Read the model definition and answer for the solid it produces. Units are mm, in the model's axes. A direction names the side the tool comes from. Give positions to 0.01 mm unless a question says otherwise; leave off trailing zeros. Loops run counter-clockwise (first coordinate to the right, second up) from the corner with the lowest first, then second, coordinate; pieces in that order, holes last. Notation, with made-up numbers: (60.25, 6) -> (80.25, 6) arc R17 cw to (80.25, 13) -> close; hole circle Ø10 at (-3, 62.5). An arc over 180 degrees is marked (long way). Write each question's results on one line, items separated by ' | '. Start each with the question number.
Item 1: Section B-B on x = 14.5 is taken. Write down the section's boundary in (y, z), and give its area (3 significant figures).
Item 2: Determine the mould class of faces 1 (the cylindrical face through (-17.198, 33.596, 6.261)), 2 (the conical face through (15.932, -27.797, 5.239)), 3 (the flat face through (0, 0, 0)) for opening direction Z: +Z half, -Z half, draft (parallel to the pull), parting line (faces both ways), or undercut.
Item 3: Which of the six approach directions +Z, -Z, +X, -X, +Y, -Y give full straight-line access (tool end or side, diameter ignored) to faces 4 (the flat face through (-26, -35, 6)), 5 (the cylindrical face through (-17, -33.5, 6.3)), 6 (the cylindrical face through (22.22, -15.463, 5.425)), 7 (the cylindrical face through (-22.22, 25.787, 5.425))?
Item 4: Section A-A on x = 21 is taken. Write down the section's boundary in (y, z).
Item 5: Each of these flat-tipped pins is pushed along its axis until it touches: P1, Ø3, axis at y = -27.5, z = 5.2, coming from the +X side; P2, Ø1.5, axis at x = -0.5, y = -13.5, coming from the -Z side; P3, Ø1.9, axis at y = -20.625, z = 5.2, coming from the -X side; P4, Ø3, axis at y = 20.625, z = 5.2, coming from the -X side. Where does it stop, or does it pass through?
Item 6: Find the intervals of material crossed by line 1 (Z direction, x = 23, y = 0); line 2 (X direction, y = 29.5, z = 6.5); line 3 (Y direction, x = -23, z = 9), in increasing order.
```python
from build123d import *

# Parameters (mm, degrees)
SKETCH1_W                           = 55
SKETCH1_H                           = 70
BOSS_EXTRUDE1_DEPTH                 = 12.7
SKETCH21_RX                         = 14
SKETCH21_RY                         = 10.5
CUT_EXTRUDE1_DEPTH                  = 47.287579328
FILLET2_START                       = -1
FILLET2_DEPTH                       = 15
F_8_32_TAPPED_HOLE1_AT_2_COUNT      = 2
F_8_32_TAPPED_HOLE1_AT_2_PITCH      = 13.75
F_8_32_TAPPED_HOLE1_AT_3_COUNT      = 2
F_8_32_TAPPED_HOLE1_AT_3_PITCH      = 27.5
F_8_32_TAPPED_HOLE1_AT_4_COUNT      = 2
F_8_32_TAPPED_HOLE1_AT_4_PITCH      = 55
F_8_32_TAPPED_HOLE1_AT_5_COUNT      = 2
F_8_32_TAPPED_HOLE1_AT_5_PITCH      = 41.25
F_1_8_0_1250_DOWEL_HOLE1_AT_2_COUNT = 2
F_1_8_0_1250_DOWEL_HOLE1_AT_2_PITCH = 41.25


with BuildPart() as part:
    # Sketch1 → Boss-Extrude1 (new body)
    with BuildSketch(Plane.XY):
        Rectangle(SKETCH1_W, SKETCH1_H)
    extrude(amount=BOSS_EXTRUDE1_DEPTH)

    # Sketch21 → Cut-Extrude1 (cut, through all)
    with BuildSketch(Plane.XY.offset(12.7)):
        with Locations((0, 35)):
            Ellipse(SKETCH21_RX, SKETCH21_RY)
        with Locations((0, -35)):
            Ellipse(SKETCH21_RX, SKETCH21_RY)
    extrude(amount=-CUT_EXTRUDE1_DEPTH, mode=Mode.SUBTRACT)

    # Fillet2: read off the stored shape, not the designer's step
    # Fillet2 outline → Fillet2 (cut)
    with BuildSketch(Plane.XY.offset(FILLET2_START)):
        with BuildLine():
            ThreePointArc((-23.533885883, 35), (-17.113783845, 33.556632687), (-11.929223863, 29.504305309))
            add(Edge.make_bspline(
                [(-14, 35), (-14, 32.032702325), (-11.929223863, 29.504305309)],
                knots=[3.141592654, 3.141592654, 3.141592654, 3.703586408, 3.703586408, 3.703586408], degree=2, weights=[1, 0.895209737, 0.865402427]))
            Line((-14, 35), (-23.533885883, 35))
        make_face()
        with BuildLine():
            add(Edge.make_bspline(
                [(11.929223863, 29.504305309), (14, 32.032702325), (14, 35)],
                knots=[5.721191552, 5.721191552, 5.721191552, 6.283185307, 6.283185307, 6.283185307], degree=2, weights=[0.865402427, 0.895209737, 1]))
            ThreePointArc((11.929223863, 29.504305309), (17.113783845, 33.556632687), (23.533885883, 35))
            Line((23.533885883, 35), (14, 35))
        make_face()
        with BuildLine():
            ThreePointArc((23.533885883, -35), (17.113783845, -33.556632687), (11.929223863, -29.504305309))
            add(Edge.make_bspline(
                [(14, -35), (14, -32.032702325), (11.929223863, -29.504305309)],
                knots=[0, 0, 0, 0.561993755, 0.561993755, 0.561993755], degree=2, weights=[1, 0.895209737, 0.865402427]))
            Line((14, -35), (23.533885883, -35))
        make_face()
        with BuildLine():
            add(Edge.make_bspline(
                [(-11.929223863, -29.504305309), (-14, -32.032702325), (-14, -35)],
                knots=[2.579598899, 2.579598899, 2.579598899, 3.141592654, 3.141592654, 3.141592654], degree=2, weights=[0.865402427, 0.895209737, 1]))
            ThreePointArc((-11.929223863, -29.504305309), (-17.113783845, -33.556632687), (-23.533885883, -35))
            Line((-23.533885883, -35), (-14, -35))
        make_face()
    extrude(amount=FILLET2_DEPTH, mode=Mode.SUBTRACT)

    # Sketch16 → #8-32 Tapped Hole1 (revolve, cut)
    with BuildSketch(Plane(origin=(27.5, -27.5, 5.2), x_dir=(0, 0, -1), z_dir=(0, 1, 0))):
        Polygon((0, 0), (0, 11.747806461), (1.7272, 10.71), (1.7272, 0), align=None)
    f_8_32_tapped_hole1 = revolve(axis=Axis((33.85, -27.5, 5.2), (-1, 0, 0)), mode=Mode.SUBTRACT)

    # #8-32 Tapped Hole1 at 2: #8-32 Tapped Hole1 ×2
    with Locations(*[(0, i * F_8_32_TAPPED_HOLE1_AT_2_PITCH, 0) for i in range(1, F_8_32_TAPPED_HOLE1_AT_2_COUNT)]):
        add(f_8_32_tapped_hole1, mode=Mode.SUBTRACT)

    # #8-32 Tapped Hole1 at 3: #8-32 Tapped Hole1 ×2
    with Locations(*[(0, i * F_8_32_TAPPED_HOLE1_AT_3_PITCH, 0) for i in range(1, F_8_32_TAPPED_HOLE1_AT_3_COUNT)]):
        add(f_8_32_tapped_hole1, mode=Mode.SUBTRACT)

    # #8-32 Tapped Hole1 at 4: #8-32 Tapped Hole1 ×2
    with Locations(*[(0, i * F_8_32_TAPPED_HOLE1_AT_4_PITCH, 0) for i in range(1, F_8_32_TAPPED_HOLE1_AT_4_COUNT)]):
        add(f_8_32_tapped_hole1, mode=Mode.SUBTRACT)

    # #8-32 Tapped Hole1 at 5: #8-32 Tapped Hole1 ×2
    with Locations(*[(0, i * F_8_32_TAPPED_HOLE1_AT_5_PITCH, 0) for i in range(1, F_8_32_TAPPED_HOLE1_AT_5_COUNT)]):
        add(f_8_32_tapped_hole1, mode=Mode.SUBTRACT)

    # Sketch20 → 1/8 (0.1250) Dowel Hole1 (revolve, cut)
    with BuildSketch(Plane(origin=(27.5, -20.625, 5.2), x_dir=(0, 0, -1), z_dir=(0, 1, 0))):
        Polygon((0, 0), (0, 4.953866233), (1.5875, 4), (1.5875, 0), align=None)
    f_1_8_0_1250_dowel_hole1 = revolve(axis=Axis((33.85, -20.625, 5.2), (-1, 0, 0)), mode=Mode.SUBTRACT)

    # 1/8 (0.1250) Dowel Hole1 at 2: 1/8 (0.1250) Dowel Hole1 ×2
    with Locations(*[(0, i * F_1_8_0_1250_DOWEL_HOLE1_AT_2_PITCH, 0) for i in range(1, F_1_8_0_1250_DOWEL_HOLE1_AT_2_COUNT)]):
        add(f_1_8_0_1250_dowel_hole1, mode=Mode.SUBTRACT)

    # Mirror1: #8-32 Tapped Hole1, 1/8 (0.1250) Dowel Hole1 across plane
    add(f_8_32_tapped_hole1.mirror(Plane(origin=(0, 0, 0), x_dir=(0, 0, 1), z_dir=(1, 0, 0))), mode=Mode.SUBTRACT)
    add(f_1_8_0_1250_dowel_hole1.mirror(Plane(origin=(0, 0, 0), x_dir=(0, 0, 1), z_dir=(1, 0, 0))), mode=Mode.SUBTRACT)

    # Mirror1 copy 1 sketch → Mirror1 copy 1 (revolve, cut)
    with BuildSketch(Plane(origin=(-27.5, -13.75, 5.2), x_dir=(0, 0, -1), z_dir=(0, 1, 0))):
        Polygon((0, 0), (0, -11.747806461), (1.7272, -10.71), (1.7272, 0), align=None)
    revolve(axis=Axis((-33.85, -13.75, 5.2), (-1, 0, 0)), mode=Mode.SUBTRACT)

    # Mirror1 copy 2 sketch → Mirror1 copy 2 (revolve, cut)
    with BuildSketch(Plane(origin=(-27.5, 0, 5.2), x_dir=(0, 0, -1), z_dir=(0, 1, 0))):
        Polygon((0, 0), (0, -11.747806461), (1.7272, -10.71), (1.7272, 0), align=None)
    revolve(axis=Axis((-33.85, 0, 5.2), (-1, 0, 0)), mode=Mode.SUBTRACT)

    # Mirror1 copy 3 sketch → Mirror1 copy 3 (revolve, cut)
    with BuildSketch(Plane(origin=(-27.5, 27.5, 5.2), x_dir=(0, 0, -1), z_dir=(0, 1, 0))):
        Polygon((0, 0), (0, -11.747806461), (1.7272, -10.71), (1.7272, 0), align=None)
    revolve(axis=Axis((-33.85, 27.5, 5.2), (-1, 0, 0)), mode=Mode.SUBTRACT)

    # Mirror1 copy 4 sketch → Mirror1 copy 4 (revolve, cut)
    with BuildSketch(Plane(origin=(-27.5, 13.75, 5.2), x_dir=(0, 0, -1), z_dir=(0, 1, 0))):
        Polygon((0, 0), (0, -11.747806461), (1.7272, -10.71), (1.7272, 0), align=None)
    revolve(axis=Axis((-33.85, 13.75, 5.2), (-1, 0, 0)), mode=Mode.SUBTRACT)

    # Mirror1 copy 5 sketch → Mirror1 copy 5 (revolve, cut)
    with BuildSketch(Plane(origin=(-27.5, 20.625, 5.2), x_dir=(0, 0, -1), z_dir=(0, 1, 0))):
        Polygon((0, 0), (0, -4.953866233), (1.5875, -4), (1.5875, 0), align=None)
    revolve(axis=Axis((-33.85, 20.625, 5.2), (-1, 0, 0)), mode=Mode.SUBTRACT)


solid = part.part
```
Findings:
1) outline: (-31.97, 0) -> (31.97, 0) -> (31.97, 12.7) -> (-31.97, 12.7) -> close | area: 812 mm2
2) face 1: draft | face 2: undercut | face 3: -Z half
3) face 4: +Z, -Z, +X, -X, -Y | face 5: +Z, -Z, -Y | face 6: +X | face 7: -X
4) outline: (-34.78, 0) -> (34.78, 0) -> (34.78, 12.7) -> (-34.78, 12.7) -> close; hole circle Ø3.45 at (-27.5, 5.2); hole circle Ø3.45 at (-13.75, 5.2); hole circle Ø3.45 at (0, 5.2); hole circle Ø3.45 at (13.75, 5.2); hole circle Ø3.45 at (27.5, 5.2)
5) P1: x = 16.65 | P2: z = 0 | P3: x = -23.12 | P4: x = -23.45
6) line 1: 0 to 3.47, 6.93 to 12.7 | line 2: -27.5 to -11.93, 11.93 to 27.5 | line 3: -34.99 to 34.99
